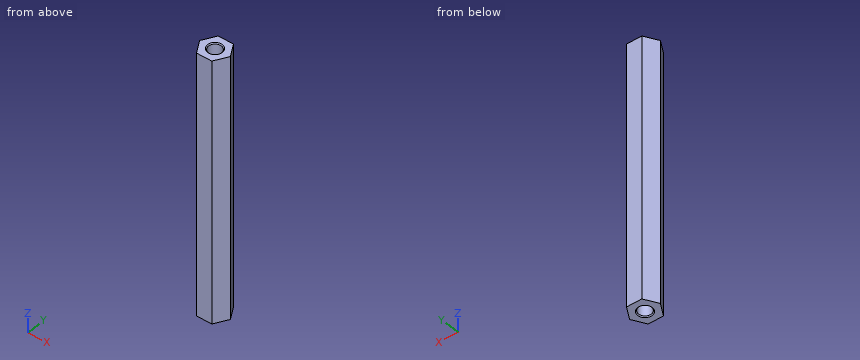
from build123d import *
from OCP.BRepFilletAPI import BRepFilletAPI_MakeChamfer

# Parameters (mm, degrees)
BOSS_EXTRUDE1_DEPTH      = 50
M2_CLEARANCE_HOLE1_D     = 2.459
M2_CLEARANCE_HOLE1_DEPTH = 11
M2_CLEARANCE_HOLE1_TIP   = 0.738758131
M2_CLEARANCE_HOLE2_D     = 2.459
M2_CLEARANCE_HOLE2_DEPTH = 11
M2_CLEARANCE_HOLE2_TIP   = 0.738758131
CHAMFER1_SIZE            = 0.000231998
CHAMFER1_SIZE2           = 0.000133944
CHAMFER2_SIZE            = 0.1705


with BuildPart() as part:
    # Sketch1 → Boss-Extrude1 (new body)
    with BuildSketch(Plane.XY.offset(25)):
        Polygon((-1.443375673, -2.5), (1.443375673, -2.5), (2.886751346, 0), (1.443375673, 2.5), (-1.443375673, 2.5), (-2.886751346, 0), align=None)
    extrude(amount=-BOSS_EXTRUDE1_DEPTH)

    # M2 Clearance Hole1
    with Locations(Plane(origin=(0, 0, -25), x_dir=(-1, 0, 0), z_dir=(0, 0, -1))):
        with Locations((0, 0)):
            Hole(M2_CLEARANCE_HOLE1_D / 2, depth=M2_CLEARANCE_HOLE1_DEPTH)
            with Locations((0, 0, -(M2_CLEARANCE_HOLE1_DEPTH + M2_CLEARANCE_HOLE1_TIP / 2))):  # 118° drill point
                Cone(0, M2_CLEARANCE_HOLE1_D / 2, M2_CLEARANCE_HOLE1_TIP, mode=Mode.SUBTRACT)

    # M2 Clearance Hole2
    with Locations(Plane.XY.offset(25)):
        with Locations((0, 0)):
            Hole(M2_CLEARANCE_HOLE2_D / 2, depth=M2_CLEARANCE_HOLE2_DEPTH)
            with Locations((0, 0, -(M2_CLEARANCE_HOLE2_DEPTH + M2_CLEARANCE_HOLE2_TIP / 2))):  # 118° drill point
                Cone(0, M2_CLEARANCE_HOLE2_D / 2, M2_CLEARANCE_HOLE2_TIP, mode=Mode.SUBTRACT)

    # Chamfer1: one chamfer whose edges measure the first distance from different faces: ONE call of the kernel's chamfer builder (chamfer() names one face for all edges)
    chamfer1_edges_1 = [part.edges().sort_by_distance(p)[0] for p in [
        (2.165063509, -1.25, -25),
        (2.165063509, 1.25, -25),
        (0, 2.5, -25),
        (-2.165063509, 1.25, -25),
        (-2.165063509, -1.25, -25),
        (0, -2.5, -25),
    ]]
    chamfer1_side_1 = [part.faces().sort_by_distance(p)[0] for p in [
        (0, -2.423623738, -25),
    ]]
    chamfer1_edges_2 = [part.edges().sort_by_distance(p)[0] for p in [
        (-2.165063509, 1.25, 25),
    ]]
    chamfer1_side_2 = [part.faces().sort_by_distance(p)[0] for p in [
        (-2.165063509, 1.25, 0),
    ]]
    chamfer1_edges_3 = [part.edges().sort_by_distance(p)[0] for p in [
        (0, 2.5, 25),
    ]]
    chamfer1_side_3 = [part.faces().sort_by_distance(p)[0] for p in [
        (0, 2.5, 0),
    ]]
    chamfer1_edges_4 = [part.edges().sort_by_distance(p)[0] for p in [
        (2.165063509, 1.25, 25),
    ]]
    chamfer1_side_4 = [part.faces().sort_by_distance(p)[0] for p in [
        (2.165063509, 1.25, 0),
    ]]
    chamfer1_edges_5 = [part.edges().sort_by_distance(p)[0] for p in [
        (2.165063509, -1.25, 25),
    ]]
    chamfer1_side_5 = [part.faces().sort_by_distance(p)[0] for p in [
        (2.165063509, -1.25, 0),
    ]]
    chamfer1_edges_6 = [part.edges().sort_by_distance(p)[0] for p in [
        (0, -2.5, 25),
    ]]
    chamfer1_side_6 = [part.faces().sort_by_distance(p)[0] for p in [
        (0, -2.5, 0),
    ]]
    chamfer1_edges_7 = [part.edges().sort_by_distance(p)[0] for p in [
        (-2.165063509, -1.25, 25),
    ]]
    chamfer1_side_7 = [part.faces().sort_by_distance(p)[0] for p in [
        (-2.165063509, -1.25, 0),
    ]]
    chamfer1 = BRepFilletAPI_MakeChamfer(part.part.solid().wrapped)
    for e in chamfer1_edges_1:
        chamfer1.Add(CHAMFER1_SIZE, CHAMFER1_SIZE2, e.wrapped, chamfer1_side_1[0].wrapped)  # the first distance lies on this face
    for e in chamfer1_edges_2:
        chamfer1.Add(CHAMFER1_SIZE, CHAMFER1_SIZE2, e.wrapped, chamfer1_side_2[0].wrapped)  # the first distance lies on this face
    for e in chamfer1_edges_3:
        chamfer1.Add(CHAMFER1_SIZE, CHAMFER1_SIZE2, e.wrapped, chamfer1_side_3[0].wrapped)  # the first distance lies on this face
    for e in chamfer1_edges_4:
        chamfer1.Add(CHAMFER1_SIZE, CHAMFER1_SIZE2, e.wrapped, chamfer1_side_4[0].wrapped)  # the first distance lies on this face
    for e in chamfer1_edges_5:
        chamfer1.Add(CHAMFER1_SIZE, CHAMFER1_SIZE2, e.wrapped, chamfer1_side_5[0].wrapped)  # the first distance lies on this face
    for e in chamfer1_edges_6:
        chamfer1.Add(CHAMFER1_SIZE, CHAMFER1_SIZE2, e.wrapped, chamfer1_side_6[0].wrapped)  # the first distance lies on this face
    for e in chamfer1_edges_7:
        chamfer1.Add(CHAMFER1_SIZE, CHAMFER1_SIZE2, e.wrapped, chamfer1_side_7[0].wrapped)  # the first distance lies on this face
    add(Compound.cast(chamfer1.Shape()), mode=Mode.REPLACE)

    # Chamfer2
    chamfer2_edges = [part.edges().sort_by_distance(p)[0] for p in [
        (-1.2295, 0, -25),
        (1.2295, 0, 25),
    ]]
    chamfer(chamfer2_edges, length=CHAMFER2_SIZE)


solid = part.part
Source: CAD feature listing. Evaluate the final solid. Frame: model axes, mm. Coordinates: 2 decimals unless noted, no trailing zeros. Loops run counter-clockwise (first coordinate to the right, second up) from the corner with the lowest first, then second, coordinate; pieces in that order, holes last. Notation, with made-up numbers: (-37, 43.5) - (-9, 43.5) arc R13 ccw to (-9, 61.5) - close; hole circle Ø3 at (-8, -29.5). An arc over 180 degrees is marked (long way). One line per item, written item: value. Start each with the question number.
1. Section B-B (z = 6). Return the cut outline in (x, y), and give its area (3 significant figures).
2. Ray query, L1, parallel to Y at x = 0, z = -16.5; L2, parallel to X at y = 0, z = -22; L3, parallel to Y at x = 0.45, z = 15. Return the intervals inside material, ascending.
3. Contact query for flat-ended pins moving along their axis: P1, Ø2, axis at y = 0.5, z = -10, coming from the -X side; P2, Ø1.5, axis at x = 0, y = 0, coming from the +Z side; P3, Ø1.5, axis at x = 0, y = 0, coming from the -Z side. Output: stop coordinate, or through.
4. Section A-A (z = 18). Return the cut outline in (x, y), and give its area (3 significant figures).
Verdict:
1. outline: (-2.89, 0) - (-1.44, -2.5) - (1.44, -2.5) - (2.89, 0) - (1.44, 2.5) - (-1.44, 2.5) - close
1. area: 21.7 mm2
2. L1: y = -2.5 to -1.23, 1.23 to 2.5
2. L2: x = -2.89 to -1.23, 1.23 to 2.89
2. L3: y = -2.5 to -1.14, 1.14 to 2.5
3. P1: stops at x = -2.89
3. P2: stops at z = 13.71
3. P3: stops at z = -13.71
4. outline: (-2.89, 0) - (-1.44, -2.5) - (1.44, -2.5) - (2.89, 0) - (1.44, 2.5) - (-1.44, 2.5) - close; hole circle Ø2.46 at (0, 0)
4. area: 16.9 mm2
